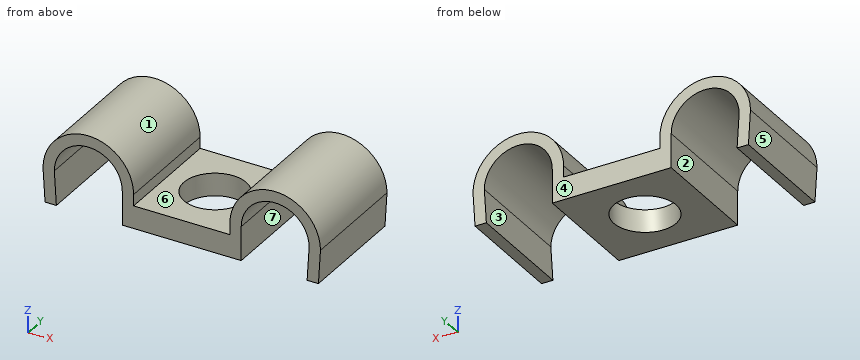
```python
from build123d import *

# Parameters (mm, degrees)
F1_DEPTH = 10
F2_R     = 2.75
F3_DEPTH = 2.5


with BuildPart() as f1:
    # F0 (on Front) → F1 (new body)
    with BuildSketch(Plane.XZ):
        with BuildLine():
            ThreePointArc((-4.25, 0), (-8.25, 4), (-12.25, 0))
            Line((-12.25, 0), (-12.069366, -3))
            Line((-12.069366, -3), (-11.069366, -3))
            Line((-11.069366, -3), (-11.25, 0))
            ThreePointArc((-11.25, 0), (-8.25, 3), (-5.25, 0))
            Line((-5.25, 0), (-5.25, -3))
            Line((-5.25, -3), (5.25, -3))
            Line((5.25, -3), (5.25, 0))
            ThreePointArc((5.25, 0), (8.25, 3), (11.25, 0))
            Line((11.25, 0), (11.069366, -3))
            Line((11.069366, -3), (12.069366, -3))
            Line((12.069366, -3), (12.25, 0))
            ThreePointArc((12.25, 0), (8.25, 4), (4.25, 0))
            Line((4.25, 0), (4.25, -1))
            Line((4.25, -1), (-4.25, -1))
            Line((-4.25, -1), (-4.25, 0))
        make_face()
    extrude(amount=F1_DEPTH)

    # F2 (on face) → F3 (cut)
    with BuildSketch(Plane.XY.offset(-1)):
        with Locations((0, -5)):
            Circle(F2_R)
    extrude(amount=-F3_DEPTH, mode=Mode.SUBTRACT)


solid = f1.part
```
Build history of the part. All positions in model axes, mm. Face numbers are marked on the shaded views. A direction names the side the tool comes from. Coordinates: 2 decimals unless noted, no trailing zeros. Order: outer loops, then holes, each group sorted by start corner. A loop starts at its lowest first (then second) coordinate and runs counter-clockwise, first axis right, second up. Notation, with made-up numbers: (5.5, 23) -> (61.5, 23) arc R22 ccw to (61.5, 55) -> close; hole circle Ø11 at (5, -9). An arc over 180 degrees is marked (long way). Answer in a Markdown table with one row per item. Add a question column.
Q1. Band-saw the part on C-C, the plane y = -6. List the corners of the cut face in (x, z), then the cut area to 3 significant figures.
Q2. Which spindle directions (+Z, -Z, +X, -X, +Y, -Y) get a long thin tool onto all of the face, cutting with end or side? Do the marked faces 1, 2 and 3. Say none if no direction does.
Q3. Drop flat-ended pins along their axis: pin 1 (3.5 mm diameter, centred on y = -6.5, z = -1, fed in from +X); pin 2 (0.5 mm diameter, centred on y = -6, z = -0.5, fed in from -X); pin 3 (2.5 mm diameter, centred on x = 2, y = -7, fed in from +Z). Give the stop position or say it passes through.
Q4. Wall check: line 1 along Y through (x, z) = (0, -1.95); line 2 along X through (y, z) = (-7.75, 1); line 3 along X through (y, z) = (-1.5, 1.5). Give the ranges that are in metal, low to high. Write a range as [from, to].
Q5. Band-saw the part on D-D, the plane y = -0.75. List the corners of the cut face in (x, z), then the cut area to 3 significant figures.
Q6. Band-saw the part on A-A, the plane x = 0. List the corners of the cut face in (y, z).
Q7. Mould opens along X. For the marked faces 4, 5, 6 and 7 say: +X half, -X half, draft (parallel to the pull), parting line (faces both ways), or undercut.
Q8. Band-saw the part on B-B, the plane z = -0.25. List the corners of the cut face in (x, y).
Answers follow:
| question | item | result |
|---|---|---|
| 1 | outline | (-12.25, 0) -> (-12.07, -3) -> (-11.07, -3) -> (-11.25, 0) arc R3 cw to (-5.25, 0) -> (-5.25, -3) -> (-2.56, -3) -> (-2.56, -1) -> (-4.25, -1) -> (-4.25, 0) arc R4 ccw to start; (2.56, -3) -> (5.25, -3) -> (5.25, 0) arc R3 cw to (11.25, 0) -> (11.07, -3) -> (12.07, -3) -> (12.25, 0) arc R4 ccw to (4.25, 0) -> (4.25, -1) -> (2.56, -1) -> close |
| 1 | area | 40.7 mm^2 |
| 2 | face 1 | +Z, +Y, -Y |
| 2 | face 2 | -Z, +Y, -Y |
| 2 | face 3 | +Y, -Y |
| 3 | pin 1 | x = 12.25 |
| 3 | pin 2 | x = -12.23 |
| 3 | pin 3 | z = -1 |
| 4 | line 1 | [-10, -7.75], [-2.25, 0] |
| 4 | line 2 | [-12.12, -11.08], [-5.42, -4.38], [4.38, 5.42], [11.08, 12.12] |
| 4 | line 3 | [-11.96, -10.85], [-5.65, -4.54], [4.54, 5.65], [10.85, 11.96] |
| 5 | outline | (-12.25, 0) -> (-12.07, -3) -> (-11.07, -3) -> (-11.25, 0) arc R3 cw to (-5.25, 0) -> (-5.25, -3) -> (5.25, -3) -> (5.25, 0) arc R3 cw to (11.25, 0) -> (11.07, -3) -> (12.07, -3) -> (12.25, 0) arc R4 ccw to (4.25, 0) -> (4.25, -1) -> (-4.25, -1) -> (-4.25, 0) arc R4 ccw to start |
| 5 | area | 51.0 mm^2 |
| 6 | outline | (-10, -3) -> (-7.75, -3) -> (-7.75, -1) -> (-10, -1) -> close; (-2.25, -3) -> (0, -3) -> (0, -1) -> (-2.25, -1) -> close |
| 7 | face 4 | draft |
| 7 | face 5 | -X half |
| 7 | face 6 | undercut |
| 7 | face 7 | undercut |
| 8 | outline | (-12.23, -10) -> (-11.23, -10) -> (-11.23, 0) -> (-12.23, 0) -> close; (-5.25, -10) -> (-4.25, -10) -> (-4.25, 0) -> (-5.25, 0) -> close; (4.25, -10) -> (5.25, -10) -> (5.25, 0) -> (4.25, 0) -> close; (11.23, -10) -> (12.23, -10) -> (12.23, 0) -> (11.23, 0) -> close |
